```python
from build123d import *

# Parameters (mm, degrees)
SKETCH_2_R               = 1
CUT_EXTRUDE_2_DEPTH      = 10
CUT_EXTRUDE_4_DEPTH      = 9.5
CHAMFER_1_SIZE           = 1
SKETCH_3_R               = 1.25
SKETCH_3_R_2             = 1.6
CUT_EXTRUDE_3_DEPTH      = 28.5
CUT_EXTRUDE_3_DEPTH_BACK = 28.5
SKETCH_7_R               = 3.25
CUT_EXTRUDE_5_DEPTH      = 23
HOLE_WIZARD_M5_1_D       = 4.2


with BuildPart() as part:
    # 草图1 → 旋转1 (revolve)
    with BuildSketch(Plane.XY):
        Polygon((-10, 2), (-27.5, 2), (-27.5, 6), (-12, 6), (-12, 15.5), (-5, 15.5), (-5, 0), (-10, 0), align=None)
    revolve(axis=Axis((0, 0, 0), (0, 1, 0)))

    # 草图2 → 切除-拉伸2 (cut)
    with BuildSketch(Plane.XZ.offset(-2)):
        with Locations((-11.25, 19.485571585)):
            Circle(SKETCH_2_R)
        with Locations((11.25, 19.485571585)):
            Circle(SKETCH_2_R)
        with Locations((22.5, 0)):
            Circle(SKETCH_2_R)
        with Locations((11.25, -19.485571585)):
            Circle(SKETCH_2_R)
        with Locations((-11.25, -19.485571585)):
            Circle(SKETCH_2_R)
        with Locations((-22.5, 0)):
            Circle(SKETCH_2_R)
    extrude(amount=-CUT_EXTRUDE_2_DEPTH, mode=Mode.SUBTRACT)

    # 草图6 → 切除-拉伸4 (cut)
    with BuildSketch(Plane.XZ.offset(-15.5)):
        with BuildLine():
            Line((11.478240283, -3.5), (-11.478240283, -3.5))
            ThreePointArc((-11.478240283, -3.5), (0, -12), (11.478240283, -3.5))
        make_face()
    extrude(amount=CUT_EXTRUDE_4_DEPTH, mode=Mode.SUBTRACT)

    # 倒角1
    chamfer_1_edges = [part.edges().sort_by_distance(p)[0] for p in [
        (0, 15.5, 12),
        (0, 6, 12),
    ]]
    chamfer(chamfer_1_edges, length=CHAMFER_1_SIZE)

    # 草图3 → 切除-拉伸3 (cut, two sides)
    with BuildSketch(Plane.XY) as cut_extrude_3_sk:
        with Locations((0, 9.5)):
            Circle(SKETCH_3_R)
        with Locations((7.5, 12)):
            Circle(SKETCH_3_R_2)
        with Locations((-7.5, 12)):
            Circle(SKETCH_3_R_2)
    extrude(amount=CUT_EXTRUDE_3_DEPTH, mode=Mode.SUBTRACT)
    extrude(cut_extrude_3_sk.sketch, amount=-CUT_EXTRUDE_3_DEPTH_BACK, mode=Mode.SUBTRACT)

    # 草图7 → 切除-拉伸5 (cut, through all)
    with BuildSketch(Plane(origin=(0, 0, 5.5), x_dir=(-1, 0, 0), z_dir=(0, 0, -1))):
        with Locations((-7.5, 12)):
            Circle(SKETCH_7_R)
        with Locations((7.5, 12)):
            Circle(SKETCH_7_R)
    extrude(amount=-CUT_EXTRUDE_5_DEPTH, mode=Mode.SUBTRACT)

    # M5 螺纹孔1 (through all)
    with Locations(Plane(origin=(0, 6, 0), x_dir=(1, 0, 0), z_dir=(0, 1, 0))):
        with Locations((11.25, 19.485571585), (22.5, 0), (11.25, -19.485571585), (-11.25, -19.485571585), (-22.5, 0), (-11.25, 19.485571585)):
            Hole(HOLE_WIZARD_M5_1_D / 2)


solid = part.part
```
CAD build for the part. Positions are in the model's coordinates, mm. A direction names the side the tool comes from. Round coordinates to 2 decimals unless told otherwise and drop trailing zeros. Loops run counter-clockwise (first coordinate to the right, second up) from the corner with the lowest first, then second, coordinate; pieces in that order, holes last. Notation, with made-up numbers: (-0.75, -17) - (34.25, -17) arc R27 ccw to (34.25, 9) - close; hole circle Ø10 at (60, 70.25). An arc over 180 degrees is marked (long way). Return JSON: item names as keys, results as strings. Group by question number.
Q1. Two-plate mould, pull along Y, no slides. Class faces 5 (the face through (-4.253, 12.132, 7.685)), 6 (the face through (2.17, 1.01, -9.76)), 7 (the face through (0.2, 15.5, 5.5)), 8 (the face through (-0.16, 10.74, 8.37)): +Y half, -Y half, draft (parallel to the pull), parting line (faces both ways), or undercut.
Q2. Tool access for faces 1 (the face through (0, 6, -6)), 2 (the face through (-7, 10, -3.5)), 3 (the face through (4.253, 11.868, 7.685)), 4 (the face through (0, 2, -12)): list every direction of +Z, -Z, +X, -X, +Y, -Y with a clear straight run to the whole face (end or side of a thin tool).
Q3. Band-saw the part on B-B on x = 0. Give the cut face in (y, z), plus the area to 3 significant figures.
Q4. Band-saw the part on D-D on y = 9.5. Give the cut face in (x, z).
Q5. Band-saw the part on C-C on y = 4.75. Give the cut face in (x, z), plus the area to 3 significant figures.
Q6. Flat gauge pins, fed straight in: pin 1 Ø5.5 at (x, z) = (-11.25, -19.49) entering from +Y; pin 2 Ø5 at (x, z) = (22.5, 0) entering from -Y; pin 3 Ø4 at (x, y) = (7.5, 12) entering from +Z; pin 4 Ø2.5 at (x, y) = (-7.5, 12) entering from -Z. Where does each tip first touch, or does it go through?
Q7. Band-saw the part on A-A on z = 0. Give the number of separate pieces and of enclosed holes in the cut face, plus the area to 3 significant figures.
Q8. Drill centre lines: line 1 along X through (y, z) = (5, -18); line 2 along X through (y, z) = (2.25, -18.5); line 3 along Y through (x, z) = (-6, 15.5). Where is each one in solid material? Low to high. Write a range as [from, to].
Solutions:
{
 "1": {"face 5": "undercut", "face 6": "draft", "face 7": "+Y half", "face 8": "undercut"},
 "2": {"face 1": "+Y", "face 2": "-Z, +X, -X, +Y", "face 3": "+Z", "face 4": "-Y"},
 "3": {"outline": "(0, -10) - (2, -10) - (2, -27.5) - (6, -27.5) - (6, -5) - (0, -5) - close; (0, 5) - (8.25, 5) - (8.25, 12) - (7, 12) - (6, 13) - (6, 27.5) - (2, 27.5) - (2, 10) - (0, 10) - close; (10.75, 5) - (15.5, 5) - (15.5, 11) - (14.5, 12) - (10.75, 12) - close", "area": "249 mm^2"},
 "4": {"outline": "(-11.48, -3.5) - (-3.57, -3.5) arc R5 cw to (-1.25, 4.84) - (-1.25, 11.93) arc R12 ccw to (-5.42, 10.7) - (-5.42, 5.5) - (-9.58, 5.5) - (-9.58, 7.23) arc R12 ccw to start; (1.25, 4.84) arc R5 cw to (3.57, -3.5) - (11.48, -3.5) arc R12 ccw to (9.58, 7.23) - (9.58, 5.5) - (5.42, 5.5) - (5.42, 10.7) arc R12 ccw to (1.25, 11.93) - close"},
 "5": {"outline": "circle Ø55 at (0, 0); hole circle Ø4.2 at (-22.5, 0); hole circle Ø4.2 at (-11.25, -19.49); hole circle Ø4.2 at (-11.25, 19.49); hole circle Ø10 at (0, 0); hole circle Ø4.2 at (11.25, -19.49); hole circle Ø4.2 at (11.25, 19.49); hole circle Ø4.2 at (22.5, 0)", "area": "2,210 mm^2"},
 "6": {"pin 1": "stops at y = 6", "pin 2": "stops at y = 2", "pin 3": "stops at z = 5.5", "pin 4": "passes through"},
 "7": {"separate pieces": "4", "enclosed holes": "2", "area": "283 mm^2"},
 "8": {"line 1": "x = [-20.79, -12.73], [-9.77, 9.77], [12.73, 20.79]", "line 2": "x = [-20.35, -13.1], [-9.4, 9.4], [13.1, 20.35]", "line 3": "y = [2, 6]"}
}
